from build123d import *

# Parameters (mm, degrees)
F0_W      = 12.7
F0_H      = 57.15
F1_DEPTH  = 12.7
F2_W      = 25.4
F2_H      = 6.35
F2_W_2    = 12.7
F3_DEPTH  = 20.32
F4_W      = 25.4
F4_H      = 6.35
F4_W_2    = 12.7
F5_DEPTH  = 50.8
F6_W      = 12.7
F6_H      = 50.8
F7_DEPTH  = 12.7
F9_DEPTH  = 12.7
F11_DEPTH = 12.7
F13_DEPTH = 12.7
F14_W     = 12.7
F14_H     = 50.8
F15_DEPTH = 12.7
F16_R     = 3.81
F18_DEPTH = 6.35
F19_R     = 3.81


# Not quite as in the source:
# - a feature names something its author has since deleted; it is built from what else it names


with BuildPart() as f1:
    # F0 (on Top) → F1 (new body)
    with BuildSketch(Plane.XY):
        Polygon((101.6, -34.925), (101.6, 34.925), (88.9, 34.925), (88.9, -22.225), (76.2, -22.225), (76.2, 34.925), (63.5, 34.925), (63.5, -22.225), (50.8, -22.225), (50.8, 34.925), (38.1, 34.925), (38.1, -22.225), (25.4, -22.225), (25.4, 34.925), (12.7, 34.925), (12.7, -22.225), (0, -22.225), (0, 34.925), (-12.7, 34.925), (-12.7, -22.225), (-25.4, -22.225), (-25.4, 34.925), (-38.1, 34.925), (-38.1, -22.225), (-50.8, -22.225), (-50.8, 34.925), (-63.5, 34.925), (-63.5, -22.225), (-76.2, -22.225), (-76.2, 34.925), (-88.9, 34.925), (-88.9, -22.225), (-101.6, -22.225), (-101.6, -34.925), align=None)
        with Locations((-95.25, 6.35)):
            Rectangle(F0_W, F0_H)
    extrude(amount=F1_DEPTH)

    # F2 (on face) → F3 (join)
    with BuildSketch(Plane.XY.offset(12.7)):
        with Locations((-88.9, -11.43)):
            Rectangle(F2_W, F2_H)
        with Locations((-31.75, -11.43)):
            Rectangle(F2_W_2, F2_H)
        with Locations((-6.35, -11.43)):
            Rectangle(F2_W_2, F2_H)
        with Locations((19.05, -11.43)):
            Rectangle(F2_W_2, F2_H)
        with Locations((44.45, -11.43)):
            Rectangle(F2_W_2, F2_H)
        with Locations((69.85, -11.43)):
            Rectangle(F2_W_2, F2_H)
        with Locations((95.25, -11.43)):
            Rectangle(F2_W_2, F2_H)
        with Locations((-57.15, -11.43)):
            Rectangle(F2_W_2, F2_H)
    extrude(amount=F3_DEPTH)

    # F4 (on face) → F5 (join)
    with BuildSketch(Plane.XY.offset(33.02)):
        with Locations((-88.9, -11.43)):
            Rectangle(F4_W, F4_H)
        with Locations((-69.85, -11.43)):
            Rectangle(F4_W_2, F4_H)
        with Locations((-57.15, -11.43)):
            Rectangle(F4_W_2, F4_H)
        with Locations((-44.45, -11.43)):
            Rectangle(F4_W_2, F4_H)
        with Locations((-31.75, -11.43)):
            Rectangle(F4_W_2, F4_H)
        with Locations((-19.05, -11.43)):
            Rectangle(F4_W_2, F4_H)
        with Locations((-6.35, -11.43)):
            Rectangle(F4_W_2, F4_H)
        with Locations((6.35, -11.43)):
            Rectangle(F4_W_2, F4_H)
        with Locations((19.05, -11.43)):
            Rectangle(F4_W_2, F4_H)
        with Locations((31.75, -11.43)):
            Rectangle(F4_W_2, F4_H)
        with Locations((44.45, -11.43)):
            Rectangle(F4_W_2, F4_H)
        with Locations((57.15, -11.43)):
            Rectangle(F4_W_2, F4_H)
        with Locations((69.85, -11.43)):
            Rectangle(F4_W_2, F4_H)
        with Locations((82.55, -11.43)):
            Rectangle(F4_W_2, F4_H)
        with Locations((95.25, -11.43)):
            Rectangle(F4_W_2, F4_H)
    extrude(amount=F5_DEPTH)

    # F6 (on face) → F7 (join)
    with BuildSketch(Plane(origin=(-101.6, 0, 0), x_dir=(0, -1, 0), z_dir=(-1, 0, 0))):
        Polygon((8.255, 63.5), (8.255, 12.7), (-4.445, 12.7), (-34.925, 12.7), (-34.925, 0), (34.925, 0), (34.925, 12.7), (14.605, 12.7), (14.605, 83.82), (8.255, 83.82), align=None)
        with Locations((1.905, 38.1)):
            Rectangle(F6_W, F6_H)
    extrude(amount=-F7_DEPTH)

    # F8 (on face) → F9 (join, through all)
    with BuildSketch(Plane.YZ.offset(-25.4)):
        Polygon((-14.605, 33.02), (-14.605, 83.82), (-34.925, 12.7), (-22.225, 12.7), (-14.605, 12.7), align=None)
    extrude(amount=-F9_DEPTH)

    # F10 (on face) → F11 (join, through all)
    with BuildSketch(Plane.YZ.offset(25.4)):
        Polygon((-14.605, 33.02), (-14.605, 83.82), (-34.925, 12.7), (-22.225, 12.7), (-14.605, 12.7), align=None)
    extrude(amount=-F11_DEPTH)

    # F12 (on face) → F13 (join, through all)
    with BuildSketch(Plane.YZ.offset(76.2)):
        Polygon((-14.605, 33.02), (-14.605, 83.82), (-34.925, 12.7), (-22.225, 12.7), (-14.605, 12.7), align=None)
    extrude(amount=-F13_DEPTH)

    # F14 (on face) → F15 (join, through all)
    with BuildSketch(Plane.YZ.offset(101.6)):
        with Locations((-1.905, 38.1)):
            Rectangle(F14_W, F14_H)
    extrude(amount=-F15_DEPTH)

    # F16
    f16_edges = [f1.edges().sort_by_distance(p)[0] for p in [
        (88.9, 34.925, 6.35),
        (63.5, 34.925, 6.35),
        (38.1, 34.925, 6.35),
        (12.7, 34.925, 6.35),
        (-12.7, 34.925, 6.35),
        (-38.1, 34.925, 6.35),
        (76.2, 34.925, 6.35),
        (50.8, 34.925, 6.35),
        (25.4, 34.925, 6.35),
        (0, 34.925, 6.35),
        (-25.4, 34.925, 6.35),
        (-50.8, 34.925, 6.35),
        (-76.2, 34.925, 6.35),
        (-63.5, 34.925, 6.35),
    ]]
    fillet(f16_edges, radius=F16_R)

    # F17 (on face) → F18 (cut, through all)
    with BuildSketch(Plane.XZ.offset(14.605)):
        Polygon((-44.45, 39.37), (-50.8, 33.02), (-38.1, 33.02), align=None)
        Polygon((-25.4, 33.02), (-12.7, 33.02), (-19.05, 39.37), align=None)
        Polygon((6.35, 39.37), (0, 33.02), (12.7, 33.02), align=None)
        Polygon((31.75, 39.37), (25.4, 33.02), (38.1, 33.02), align=None)
        Polygon((57.15, 39.37), (50.8, 33.02), (63.5, 33.02), align=None)
        Polygon((76.2, 33.02), (88.9, 33.02), (82.55, 39.37), align=None)
        Polygon((-76.2, 33.02), (-63.5, 33.02), (-69.85, 39.37), align=None)
    extrude(amount=-F18_DEPTH, mode=Mode.SUBTRACT)

    # F19
    f19_edges = [f1.edges().sort_by_distance(p)[0] for p in [
        (-88.9, 4.445, 38.1),
        (88.9, 4.445, 38.1),
    ]]
    fillet(f19_edges, radius=F19_R)


solid = f1.part
The model under review builds one solid part; all positions refer to its coordinate system, in mm. A direction names the side the tool comes from. Give positions to 0.01 mm unless a question says otherwise; leave off trailing zeros. Order: outer loops, then holes, each group sorted by start corner. A loop starts at its lowest first (then second) coordinate and runs counter-clockwise, first axis right, second up. Notation, with made-up numbers: (16.25, -2.5) -> (30.25, -2.5) arc R26 cw to (30.25, 31.5) -> close; hole circle Ø5 at (59, 70). An arc over 180 degrees is marked (long way). Write item = value, one per line. Start each with the question number.
(1) Take a section at C-C (z = 45.5). Write out the cut boundary in (x, y) (3 decimals).
(2) For L1, parallel to X at y = -31.5, z = 13; L2, parallel to X at y = -7, z = 44.5; L3, parallel to Y at x = 2.5, z = 71.5 (3 decimals), list the stretches that pass through material, from the lowest coordinate up. Write a range as from..to.
(3) For pin 1 Ø4 at (x, z) = (-72, 6.5) entering from +Y (3 decimals); pin 2 Ø2 at (x, z) = (-35, 47) entering from -Y; pin 3 Ø2 at (x, z) = (-66.5, 45.5) entering from +Y (3 decimals), all flat-tipped, find the tip position at first contact; note any pin that passes through.
(4) Tool access review of faces 3 (the flat face through (12.7, -9, 23)), 4 (the flat face through (95, -2, 63.5)), 5 (the flat face through (19, 14, 12.7)), 6 (the cylindrical face through (-51.886, 33.779, 6.439)): name each direction out of +Z, -Z, +X, -X, +Y, -Y from which nothing blocks a thin tool from reaching the whole face with its end or side.
(5) Draft analysis for pull direction X (two halves, no side actions). For faces 1 (the flat face through (88.9, -2, 25)), 2 (the flat face through (-91, 34.925, 6)), state which applies: +X half, -X half, draft (parallel to the pull), parting line (faces both ways), or undercut.
(6) Take a section at A-A (x = -23.5). Write out the cut boundary in (y, z) (3 decimals).
(7) Take a section at B-B (y = -4). State how many separate pieces and enclosed holes the cut face has, plus the area to 3 significant figures.
Returned:
q1.outline = (-101.6, -14.605) -> (-38.1, -14.605) -> (-38.1, -25.554) -> (-25.4, -25.554) -> (-25.4, -14.605) -> (12.7, -14.605) -> (12.7, -25.554) -> (25.4, -25.554) -> (25.4, -14.605) -> (63.5, -14.605) -> (63.5, -25.554) -> (76.2, -25.554) -> (76.2, -14.605) -> (101.6, -14.605) -> (101.6, 4.445) -> (92.71, 4.445) arc R3.81 ccw to (88.9, 0.635) -> (88.9, -8.255) -> (-88.9, -8.255) -> (-88.9, 0.635) arc R3.81 ccw to (-92.71, 4.445) -> (-101.6, 4.445) -> close
q2.L1 = -38.1..-25.4, 12.7..25.4, 63.5..76.2
q2.L2 = -101.6..-88.9, 88.9..101.6
q2.L3 = -14.605..-8.255
q3.pin_1 = -22.225
q3.pin_2 = -25.41
q3.pin_3 = -8.255
q4.face_3 = none
q4.face_4 = +Z, +X, -X, +Y
q4.face_5 = +Z, +Y
q4.face_6 = +Z, -Z, +Y
q5.face_1 = undercut
q5.face_2 = draft
q6.outline = (-34.925, 0) -> (-22.225, 0) -> (-22.225, 12.7) -> (-34.925, 12.7) -> close; (-14.605, 34.92) -> (-8.255, 34.92) -> (-8.255, 83.82) -> (-14.605, 83.82) -> close
q7.separate_pieces = 8
q7.enclosed_holes = 0
q7.area = 2,740 mm²
